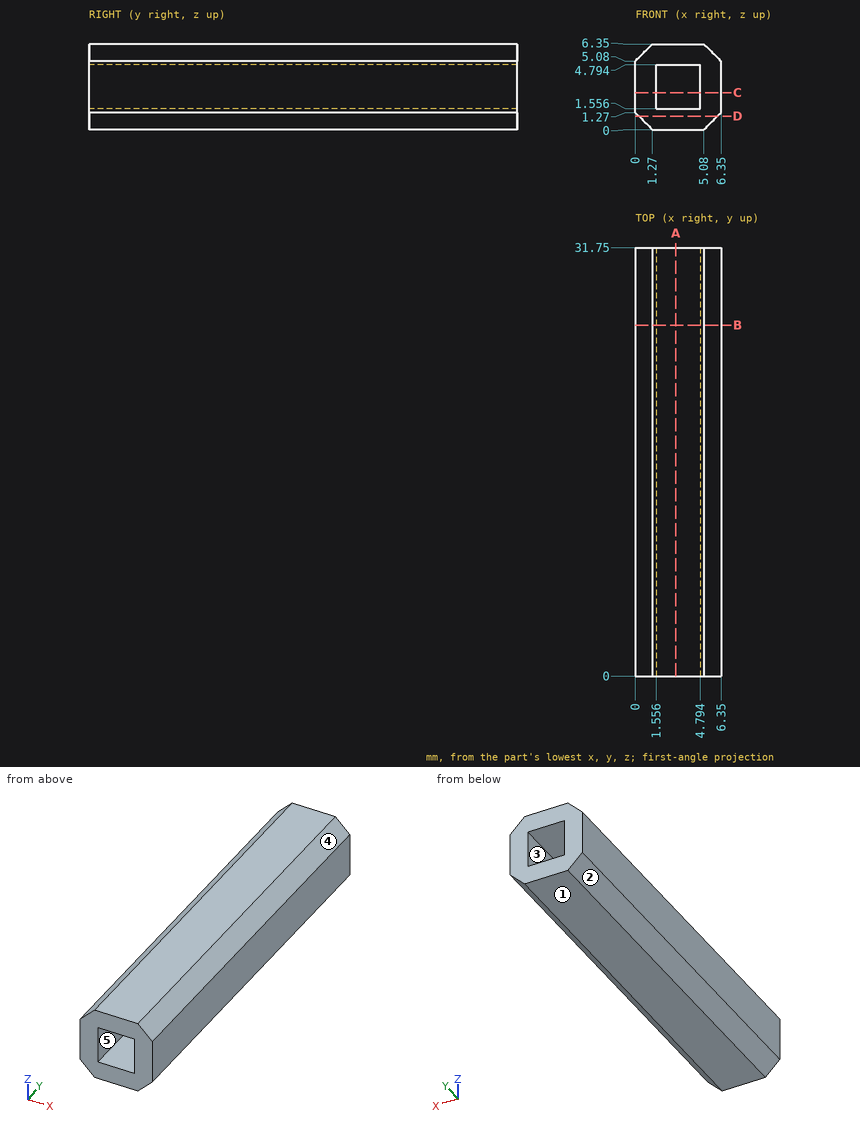
Here's the drawing with two shaded views (mm, measured from the low corner). I have some questions. A direction names the side the tool comes from. Round coordinates to 2 decimals unless told otherwise and drop trailing zeros. Write each loop counter-clockwise with the first axis right and the second up, starting at its lowest first coordinate (ties: lowest second). Pieces come first, ordered by that corner, then holes. Notation, with made-up numbers: M -27.5,-3 L 24.5,-3 A23 ccw 24.5,20 Z; hole C 22,71.5 d1. An arc over 180 degrees is marked long. Answer in a Markdown table with one row per item. Add a question column.
Q1. On a 3-axis mill with a long thin cutter (end or side, diameter ignored), from which of +Z, -Z, +X, -X, +Y, -Y can I reach the whole of each face in a straight line? I mean the marked faces 4 and 5. Say none if no direction works.
Q2. Imagine slicing it at B-B (y = 26). Please give me the cut outline in (x, z).
Q3. If I drill on line 1 (Z direction, x = 3.25, y = 12); line 2 (X direction, y = 4.5, z = 0.5), over which ranges is the centre line in solid material (lowest first)? Write a range as from..to.
Q4. If we mould it in two halves opening along X, with no side actions, what happens to the marked faces 1, 2 and 3? For each: +X half, -X half, draft (parallel to the pull), parting line (faces both ways), or undercut.
Q5. Imagine slicing it at C-C (z = 2.75). Please give me the cut outline in (x, y).
Q6. Imagine slicing it at D-D (z = 1). Please give me the cut outline in (x, y).
Q7. Imagine slicing it at A-A (x = 3). Please give me the cut outline in (y, z).
Values:
| question | item | result |
|---|---|---|
| 1 | face 4 | +Z, +X, +Y, -Y |
| 1 | face 5 | +Y, -Y |
| 2 | outline | M 0,1.27 L 1.27,0 L 5.08,0 L 6.35,1.27 L 6.35,5.08 L 5.08,6.35 L 1.27,6.35 L 0,5.08 Z; hole M 1.56,1.56 L 4.79,1.56 L 4.79,4.79 L 1.56,4.79 Z |
| 3 | line 1 | 0..1.56, 4.79..6.35 |
| 3 | line 2 | 0.77..5.58 |
| 4 | face 1 | draft |
| 4 | face 2 | -X half |
| 4 | face 3 | undercut |
| 5 | outline | M 0,0 L 1.56,0 L 1.56,31.75 L 0,31.75 Z; M 4.79,0 L 6.35,0 L 6.35,31.75 L 4.79,31.75 Z |
| 6 | outline | M 0.27,0 L 6.08,0 L 6.08,31.75 L 0.27,31.75 Z |
| 7 | outline | M 0,0 L 31.75,0 L 31.75,1.56 L 0,1.56 Z; M 0,4.79 L 31.75,4.79 L 31.75,6.35 L 0,6.35 Z |
